Check sheet for the modelled part. Datum: model origin and axes. Units: mm. Face numbers are marked on the shaded views. A direction names the side the tool comes from. Coordinates: 2 decimals unless noted, no trailing zeros. Loops run counter-clockwise (first coordinate to the right, second up) from the corner with the lowest first, then second, coordinate; pieces in that order, holes last. Notation, with made-up numbers: (40, 49.25) -> (99, 49.25) arc R20 ccw to (99, 85.25) -> close; hole circle Ø6 at (5, 47). An arc over 180 degrees is marked (long way). Use one line per item in the form item = value.
from build123d import *

# Parameters (mm, degrees)
SKIZZE2_R                       = 24.795
AUFSATZ_LINEAR_AUSTRAGEN1_DEPTH = 63.87
SKIZZE8_W                       = 20
SKIZZE8_H                       = 27.38
SCHNITT_LINEAR_AUSTRAGEN1_DEPTH = 4.4
KREISMUSTER1_COUNT              = 2
FASE1_SIZE                      = 1


with BuildPart() as part:
    # Skizze1 → Rotation1 (revolve)
    with BuildSketch(Plane(origin=(0, 0, 0), x_dir=(1, 0, 0), z_dir=(0, 1, 0)), mode=Mode.PRIVATE) as rotation1_sk:
        Polygon((-46, 0), (-46, 15.4), (0, 20.905), (0, 0), align=None)
    revolve(rotation1_sk.sketch.rotate(Axis((-46, 0, 0), (1, 0, 0)), 180), axis=Axis((-46, 0, 0), (1, 0, 0)))  # turned: the seam where the file's is

    # Skizze2 → Aufsatz-Linear austragen1 (add)
    with BuildSketch(Plane(origin=(0, 0, 0), x_dir=(0, 0, -1), z_dir=(1, 0, 0))):
        Circle(SKIZZE2_R)
    extrude(amount=AUFSATZ_LINEAR_AUSTRAGEN1_DEPTH)

    # Skizze8 → Schnitt-Linear austragen1 (cut)
    with BuildSketch(Plane(origin=(0, 24.795, 0), x_dir=(1, 0, 0), z_dir=(0, 1, 0))):
        with Locations((19.68, 0)):
            Rectangle(SKIZZE8_W, SKIZZE8_H)
    schnitt_linear_austragen1 = extrude(amount=-SCHNITT_LINEAR_AUSTRAGEN1_DEPTH, mode=Mode.SUBTRACT)

    # Kreismuster1: Schnitt-Linear austragen1 ×2 about axis
    kreismuster1_axis = Axis((0, 0, 0), (1, 0, 0))
    for i in range(1, KREISMUSTER1_COUNT):
        add(schnitt_linear_austragen1.rotate(kreismuster1_axis, i * 360 / KREISMUSTER1_COUNT), mode=Mode.SUBTRACT)

    # Fase1
    fase1_edges = [part.edges().sort_by_distance(p)[0] for p in [
        (0, 0, 24.795),
        (63.87, 0, 24.795),
    ]]
    chamfer(fase1_edges, length=FASE1_SIZE)


solid = part.part
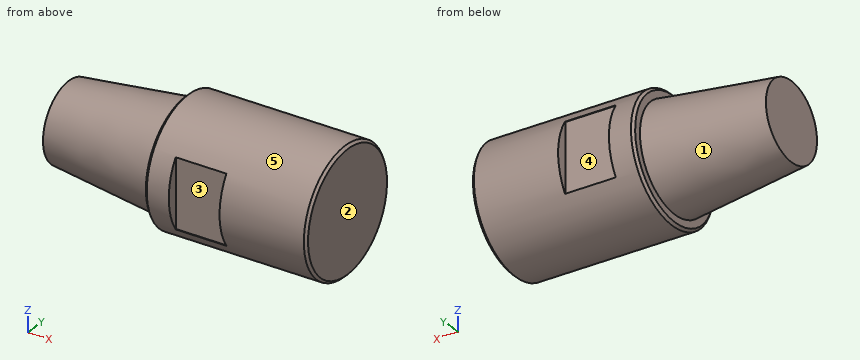
(1) Go/stop test with flat-tipped pins: P1, Ø8, axis at x = 14.5, y = -10.5, coming from the -Z side; P2, Ø4, axis at x = -9, y = -18, coming from the +Z side; P3, Ø10, axis at x = 15.5, z = 2, coming from the +Y side (3 decimals); P4, Ø10, axis at y = -14.5, z = 10, coming from the -X side. Record where each tip stops, or that it passes through.
Established:
P1 = -23.93
P2 = 11.74
P3 = 20.395
P4 = -46
(2) Mould release check, pull along Z, two halves, no side actions. Record for the marked faces 1, 2 and 3: +Z half, -Z half, draft (parallel to the pull), parting line (faces both ways), or undercut.
Established:
face_1 = parting line
face_2 = draft
face_3 = undercut
(3) Scan lines: line 1 along Z through (x, y) = (21, 7); line 2 along X through (y, z) = (16.5, -13); line 3 along Z through (x, y) = (29, -16.5). Record each from-to range of solid material in increasing order.
Established:
line_1 = -23.79 to 23.79
line_2 = 0 to 63.87
line_3 = -18.51 to 18.51
(4) Section check C-C, the plane z = 0. Record the boundary of the cut face in (x, y) (3 decimals), plus the area to 3 significant figures.
Established:
outline = (-46, -15.4) -> (0, -20.905) -> (0, -23.795) -> (1, -24.795) -> (9.68, -24.795) -> (9.68, -20.395) -> (29.68, -20.395) -> (29.68, -24.795) -> (62.87, -24.795) -> (63.87, -23.795) -> (63.87, 23.795) -> (62.87, 24.795) -> (29.68, 24.795) -> (29.68, 20.395) -> (9.68, 20.395) -> (9.68, 24.795) -> (1, 24.795) -> (0, 23.795) -> (0, 20.905) -> (-46, 15.4) -> close
area = 4,660 mm²
(5) Section check D-D, the plane x = 46.5. Record the boundary of the cut face in (y, z) (3 decimals).
Established:
outline = circle Ø49.59 at (0, 0)
(6) Section check A-A, the plane y = 0. Record the boundary of the cut face in (x, z) (3 decimals).
Established:
outline = (-46, -15.4) -> (0, -20.905) -> (0, -23.795) -> (1, -24.795) -> (62.87, -24.795) -> (63.87, -23.795) -> (63.87, 23.795) -> (62.87, 24.795) -> (1, 24.795) -> (0, 23.795) -> (0, 20.905) -> (-46, 15.4) -> close
(7) Section check B-B, the plane x = 16. Record the boundary of the cut face in (y, z) (3 decimals), plus the area to 3 significant figures.
Established:
outline = (-20.673, -13.69) arc R24.795 ccw to (20.673, -13.69) -> (20.395, -13.69) -> (20.395, 13.69) -> (20.673, 13.69) arc R24.795 ccw to (-20.673, 13.69) -> (-20.395, 13.69) -> (-20.395, -13.69) -> close
area = 1,760 mm²
(8) Tool access check on the marked faces 4 and 5. Record the directions out of +Z, -Z, +X, -X, +Y, -Y that give a thin tool (end or side, any length) a straight path to the whole face; none if there is none.
Established:
face_4 = +Y
face_5 = +X, -X
